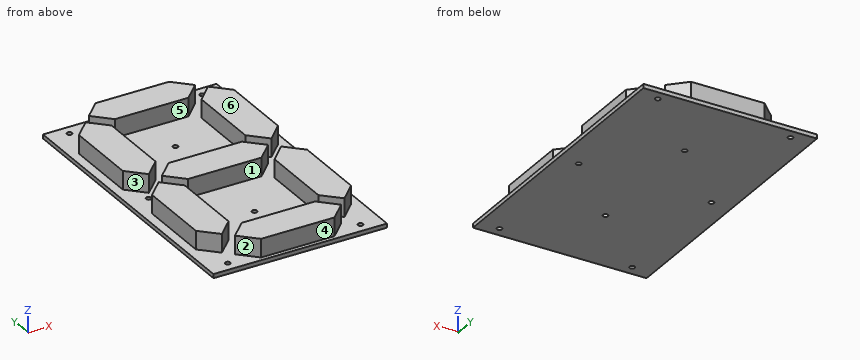
```python
from build123d import *

# Parameters (mm, degrees)
CROQUIS1_W              = 85
CROQUIS1_H              = 140
CROQUIS1_R              = 1.25
SALIENTE_EXTRUIR1_DEPTH = 2
SALIENTE_EXTRUIR2_DEPTH = 9


with BuildPart() as part:
    # Croquis1 → Saliente-Extruir1 (new body)
    with BuildSketch(Plane.XY):
        Rectangle(CROQUIS1_W, CROQUIS1_H)
        with Locations((-32.5, 65)):
            Circle(CROQUIS1_R, mode=Mode.SUBTRACT)
        with Locations((32.5, 65)):
            Circle(CROQUIS1_R, mode=Mode.SUBTRACT)
        with Locations((-32.5, 0)):
            Circle(CROQUIS1_R, mode=Mode.SUBTRACT)
        with Locations((32.5, 0)):
            Circle(CROQUIS1_R, mode=Mode.SUBTRACT)
        with Locations((-32.5, -65)):
            Circle(CROQUIS1_R, mode=Mode.SUBTRACT)
        with Locations((32.5, -65)):
            Circle(CROQUIS1_R, mode=Mode.SUBTRACT)
        with Locations((0, -32.5)):
            Circle(CROQUIS1_R, mode=Mode.SUBTRACT)
        with Locations((0, 32.5)):
            Circle(CROQUIS1_R, mode=Mode.SUBTRACT)
    extrude(amount=SALIENTE_EXTRUIR1_DEPTH)

    # Croquis2 → Saliente-Extruir2 (add)
    with BuildSketch(Plane.XY.offset(2)):
        Polygon((22, 48), (30, 56), (38, 48), (38, 12), (30, 4), (22, 12), align=None)
        Polygon((-22, 48), (-30, 56), (-38, 48), (-38, 12), (-30, 4), (-22, 12), align=None)
        Polygon((22, -48), (30, -56), (38, -48), (38, -12), (30, -4), (22, -12), align=None)
        Polygon((-22, -48), (-30, -56), (-38, -48), (-38, -12), (-30, -4), (-22, -12), align=None)
        Polygon((-18, -8), (-26, 0), (-18, 8), (18, 8), (26, 0), (18, -8), align=None)
        Polygon((-18.000001585, 52.000001585), (-26.000001585, 60.000001585), (-18.000001585, 68.000001585), (17.999998415, 68.000001585), (25.999998415, 60.000001585), (17.999998415, 52.000001585), align=None)
        Polygon((-18.000001585, -52.000001585), (-26.000001585, -60.000001585), (-18.000001585, -68.000001585), (17.999998415, -68.000001585), (25.999998415, -60.000001585), (17.999998415, -52.000001585), align=None)
    extrude(amount=SALIENTE_EXTRUIR2_DEPTH)


solid = part.part
```
Model file for the job. Use its own axes, mm. Face numbers are marked on the shaded views. A direction names the side the tool comes from. Give positions to 0.01 mm unless a question says otherwise; leave off trailing zeros. Write each loop counter-clockwise with the first axis right and the second up, starting at its lowest first coordinate (ties: lowest second). Pieces come first, ordered by that corner, then holes. Notation, with made-up numbers: (30.5, 77.5) -> (64.5, 77.5) arc R23 ccw to (64.5, 113.5) -> close; hole circle Ø1 at (54, -32.75). An arc over 180 degrees is marked (long way). Use CSV: the item, a comma, the result in double quotes. Start each with the question number.
1) Pin check, flat tips, straight feed: P1, Ø2.5, axis at x = 6, z = 7, coming from the +Y side; P2, Ø2.5, axis at y = 25, z = 8, coming from the -X side; P3, Ø2, axis at x = -29.5, z = 8, coming from the -Y side; P4, Ø2, axis at x = -32.5, y = 0, coming from the -Z side. Stop position of each tip, or through.
2) Cut at B-B on x = 3. List the corners of the cut face in (y, z), plus the area to 3 significant figures.
3) Cut at A-A on y = -27. List the corners of the cut face in (x, z), plus the area to 3 significant figures.
4) Cut at D-D on y = -49.5. List the corners of the cut face in (x, z), plus the area to 3 significant figures.
5) Cut at C-C on z = 7.75. Count the separate pieces of the cut face and the enclosed holes in it, plus the area to 3 significant figures.
6) Drill centre lines: L1, parallel to Y at x = -7, z = 4.75; L2, parallel to X at y = -65, z = 1.1; L3, parallel to Y at x = 0, z = 0.65. Where is each one in solid material? Low to high.
7) Two-plate mould, pull along Y, no slides. Class the marked faces 4, 5 and 6: released by +Y, released by -Y, zero draft, split by the parting line, or undercut.
8) Tool access for the marked faces 1, 2 and 3: list every direction of +Z, -Z, +X, -X, +Y, -Y with a clear straight run to the whole face (end or side of a thin tool).
Final values:
1,P1,"stops at y = 68"
1,P2,"stops at x = -38"
1,P3,"stops at y = -56"
1,P4,"passes through"
2,outline,"(-70, 0) -> (70, 0) -> (70, 2) -> (68, 2) -> (68, 11) -> (52, 11) -> (52, 2) -> (8, 2) -> (8, 11) -> (-8, 11) -> (-8, 2) -> (-52, 2) -> (-52, 11) -> (-68, 11) -> (-68, 2) -> (-70, 2) -> close"
2,area,"712 mm2"
3,outline,"(-42.5, 0) -> (42.5, 0) -> (42.5, 2) -> (38, 2) -> (38, 11) -> (22, 11) -> (22, 2) -> (-22, 2) -> (-22, 11) -> (-38, 11) -> (-38, 2) -> (-42.5, 2) -> close"
3,area,"458 mm2"
4,outline,"(-42.5, 0) -> (42.5, 0) -> (42.5, 2) -> (36.5, 2) -> (36.5, 11) -> (23.5, 11) -> (23.5, 2) -> (-23.5, 2) -> (-23.5, 11) -> (-36.5, 11) -> (-36.5, 2) -> (-42.5, 2) -> close"
4,area,"404 mm2"
5,separate pieces,"7"
5,enclosed holes,"0"
5,area,"4,930 mm2"
6,L1,"y = -68 to -52, -8 to 8, 52 to 68"
6,L2,"x = -42.5 to -33.75, -31.25 to 31.25, 33.75 to 42.5"
6,L3,"y = -70 to -33.75, -31.25 to 31.25, 33.75 to 70"
7,face 4,"released by -Y"
7,face 5,"undercut"
7,face 6,"zero draft"
8,face 1,"+Z"
8,face 2,"+Z, -X, -Y"
8,face 3,"+Z, -X"
